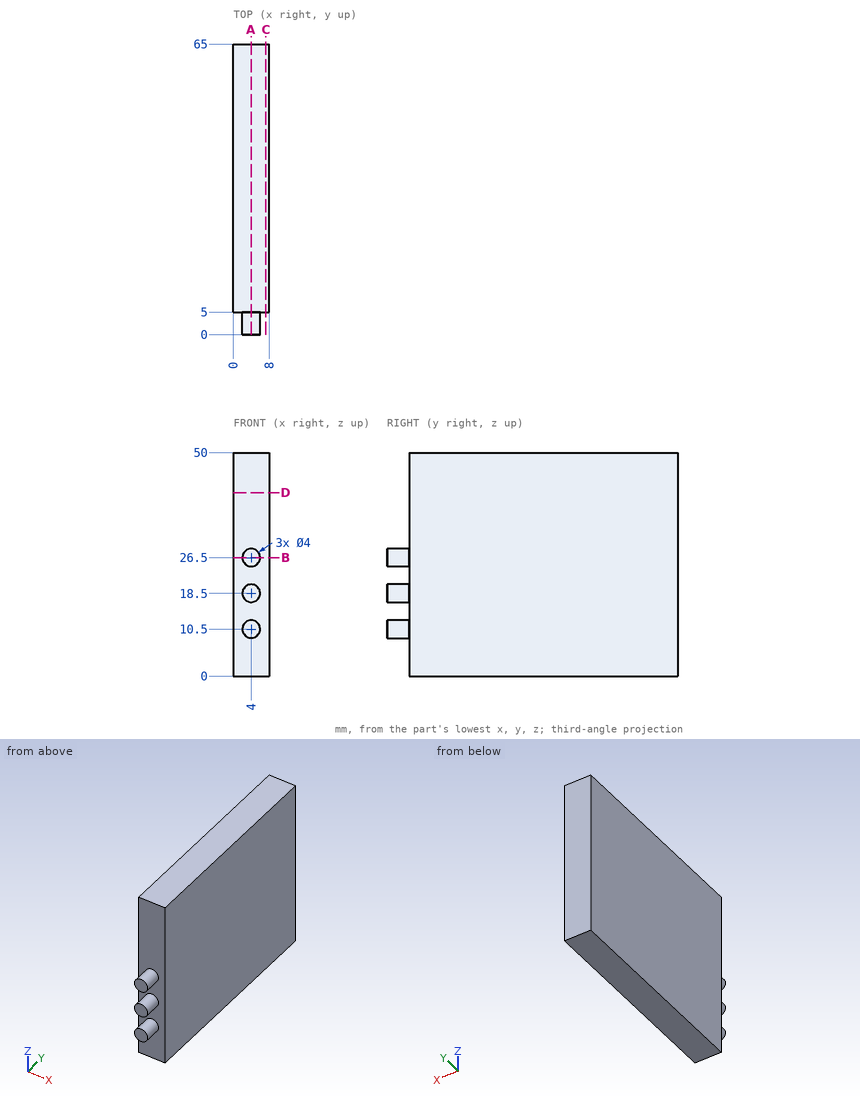
Answer from the drawing. Dimensions are ordinates in mm from the lowest x, y and z of the part. Coordinates: 2 decimals unless noted, no trailing zeros. Write each loop counter-clockwise with the first axis right and the second up, starting at its lowest first coordinate (ties: lowest second). Pieces come first, ordered by that corner, then holes. Notation, with made-up numbers: M 57.25,59 L 86.25,59 A24 cw 86.25,83 Z; hole C 57.25,52.25 d11. An arc over 180 degrees is marked long. Use a Markdown table: item, result.
Q1. A straight line is drawn through the part: L1, parallel to Y at x = 2.25, z = 40.5. Find the intervals that lie inside material, in ascending order. Write a range as [from, to].
Answer block:
| item | result |
|---|---|
| L1 | y = [5, 65] |
Q2. The part is cut by section C-C, the plane x = 7.25. Write down the section's boundary in (y, z).
Answer block:
| item | result |
|---|---|
| outline | M 5,0 L 65,0 L 65,50 L 5,50 Z |
Q3. The part is cut by section D-D, the plane z = 41. Write down the section's boundary in (x, y).
Answer block:
| item | result |
|---|---|
| outline | M 0,5 L 8,5 L 8,65 L 0,65 Z |
Q4. The part is cut by section A-A, the plane x = 4. Write down the section's boundary in (y, z), then the cut area to 3 significant figures.
Answer block:
| item | result |
|---|---|
| outline | M 0,8.5 L 5,8.5 L 5,0 L 65,0 L 65,50 L 5,50 L 5,28.5 L 0,28.5 L 0,24.5 L 5,24.5 L 5,20.5 L 0,20.5 L 0,16.5 L 5,16.5 L 5,12.5 L 0,12.5 Z |
| area | 3,060 mm2 |
Q5. This flat-tipped pin is pushed along its axis until it touches: pin 1 Ø1.5 at (x, z) = (6, 24) entering from -Y. Where does it stop, or does it pass through?
Answer block:
| item | result |
|---|---|
| pin 1 | stops at y = 5 |
Q6. The part is cut by section B-B, the plane z = 26.5. Write down the section's boundary in (x, y), then the cut area to 3 significant figures.
Answer block:
| item | result |
|---|---|
| outline | M 0,5 L 2,5 L 2,0 L 6,0 L 6,5 L 8,5 L 8,65 L 0,65 Z |
| area | 500 mm2 |
